```python
from build123d import *

# Parameters (mm, degrees)
SKETCH1_R           = 3.175
BOSS_EXTRUDE1_DEPTH = 2.54
SKETCH2_R           = 3.937
SKETCH2_R_2         = 3.175
BOSS_EXTRUDE2_DEPTH = 0.762


with BuildPart() as part:
    # Sketch1 → Boss-Extrude1 (new body)
    with BuildSketch(Plane(origin=(0, 0, 0), x_dir=(0, 0, -1), z_dir=(1, 0, 0))):
        with BuildLine():
            Line((5.08, 7.62), (5.08, -7.62))
            ThreePointArc((5.08, -7.62), (0, -12.7), (-5.08, -7.62))
            Line((-5.08, -7.62), (-5.08, 7.62))
            ThreePointArc((-5.08, 7.62), (0, 12.7), (5.08, 7.62))
        make_face()
        Circle(SKETCH1_R, mode=Mode.SUBTRACT)
    extrude(amount=BOSS_EXTRUDE1_DEPTH)

    # Sketch2 → Boss-Extrude2 (add)
    with BuildSketch(Plane(origin=(2.54, 0, 0), x_dir=(0, 0, -1), z_dir=(1, 0, 0))):
        with Locations(Location((0, 0, 0), (0, 0, 180))):
            Circle(SKETCH2_R)
        Circle(SKETCH2_R_2, mode=Mode.SUBTRACT)
    extrude(amount=BOSS_EXTRUDE2_DEPTH)


solid = part.part
```
Read the model definition and answer for the solid it produces. Units are mm, in the model's axes. A direction names the side the tool comes from. Coordinates: 2 decimals unless noted, no trailing zeros. Write each loop counter-clockwise with the first axis right and the second up, starting at its lowest first coordinate (ties: lowest second). Pieces come first, ordered by that corner, then holes. Notation, with made-up numbers: (48.5, 57) - (81.5, 57) arc R29 ccw to (81.5, 84) - close; hole circle Ø8 at (21, 35.5). An arc over 180 degrees is marked (long way). Answer as a JSON object with one key per item and string values. Group by question number.
1. A cutting plane is placed at A-A (z = 0). Determine the outline of the cut face in (x, y) (3 decimals), plus the area to 3 significant figures.
2. Which of the six approach directions +Z, -Z, +X, -X, +Y, -Y give full straight-line access (tool end or side, diameter ignored) to faces 4 (the cylindrical face through (2.916, 3.843, -0.853)), 5 (the flat face through (0, 0.2, -3.5))?
3. The mould has two halves that part along Z. Classify faces 1 (the cylindrical face through (1.63, -3.1, 0.69)), 2 (the flat face through (1, 0, -5.08)), 3 (the cylindrical face through (1.3, -12.7, -0.1)): +Z half, -Z half, draft (parallel to the pull), parting line (faces both ways), or undercut.
4. A cutting plane is placed at C-C (x = 1.75). Determine the outline of the cut face in (y, z) (3 decimals), plus the area to 3 significant figures.
5. A cutting plane is placed at B-B (y = 0). Determine the outline of the cut face in (x, z) (3 decimals), plus the area to 3 significant figures.
6. Consider L1, parallel to Y at x = 1.05, z = 0 (3 decimals); L2, parallel to Y at x = 0.2, z = -2.75; L3, parallel to X at y = -10.75, z = 2.5. Determine where each line is inside the solid, lowest interval first. Write a range as [from, to].
7. A cutting plane is placed at D-D (z = 3.5). Determine the outline of the cut face in (x, y), plus the area to 3 significant figures.
8. Each of these flat-tipped pins is pushed along its axis until it touches: P1, Ø1.5, axis at y = 0.5, z = 1.5, coming from the -X side; P2, Ø5, axis at y = -4, z = 0, coming from the +X side; P3, Ø6, axis at y = 8, z = 2.5, coming from the +X side. Where does it stop, or does it pass through?
Worked out:
{
 "1": {"outline": "(0, -12.7) - (2.54, -12.7) - (2.54, -3.937) - (3.302, -3.937) - (3.302, -3.175) - (0, -3.175) - close; (0, 3.175) - (3.302, 3.175) - (3.302, 3.937) - (2.54, 3.937) - (2.54, 12.7) - (0, 12.7) - close", "area": "49.5 mm²"},
 "2": {"face 4": "+X", "face 5": "+Z, -Z, -X, +Y, -Y"},
 "3": {"face 1": "undercut", "face 2": "-Z half", "face 3": "parting line"},
 "4": {"outline": "(-7.62, -5.08) - (7.62, -5.08) arc R5.08 ccw to (7.62, 5.08) - (-7.62, 5.08) arc R5.08 ccw to start; hole circle Ø6.35 at (0, 0)", "area": "204 mm²"},
 "5": {"outline": "(0, -5.08) - (2.54, -5.08) - (2.54, -3.937) - (3.302, -3.937) - (3.302, -3.175) - (0, -3.175) - close; (0, 3.175) - (3.302, 3.175) - (3.302, 3.937) - (2.54, 3.937) - (2.54, 5.08) - (0, 5.08) - close", "area": "10.8 mm²"},
 "6": {"L1": "y = [-12.7, -3.175], [3.175, 12.7]", "L2": "y = [-11.89, -1.59], [1.59, 11.89]", "L3": "x = [0, 2.54]"},
 "7": {"outline": "(0, -11.3) - (2.54, -11.3) - (2.54, -1.8) - (3.3, -1.8) - (3.3, 1.8) - (2.54, 1.8) - (2.54, 11.3) - (0, 11.3) - close", "area": "60.2 mm²"},
 "8": {"P1": "passes through", "P2": "stops at x = 3.3", "P3": "stops at x = 2.54"}
}
